```python
from build123d import *

# Parameters (mm, degrees)
F0_R     = 5
F1_DEPTH = 5
F0_R_2   = 10
F2_DEPTH = 15
F3_DEPTH = 10
F4_DEPTH = 5
F5_DEPTH = 20
F6_DEPTH = 10


with BuildPart() as f1:
    # F0 (on Front) → F1 (new body)
    with BuildSketch(Plane.XZ):
        with BuildLine():
            ThreePointArc((-20, 0), (-22.9289321881, 7.0710678119), (-30, 10))
            ThreePointArc((-30, 10), (-40, 0), (-30, -10))
            ThreePointArc((-30, -10), (-22.9289321881, -7.0710678119), (-20, 0))
        make_face()
        with Locations((-30, 0)):
            Circle(F0_R, mode=Mode.SUBTRACT)
    extrude(amount=F1_DEPTH)



with BuildPart() as f2:
    # F0 (on Front) → F2 (new body)
    with BuildSketch(Plane.XZ):
        with BuildLine():
            ThreePointArc((0, -15), (10.6066017178, -10.6066017178), (15, 0))
            ThreePointArc((15, 0), (10.6066017178, 10.6066017178), (0, 15))
            Line((0, 15), (-4.8648648649, 14.1891891892))
            ThreePointArc((-4.8648648649, 14.1891891892), (-15, 0), (-4.8648648649, -14.1891891892))
            Line((-4.8648648649, -14.1891891892), (0, -15))
        make_face()
        Circle(F0_R_2, mode=Mode.SUBTRACT)
    extrude(amount=F2_DEPTH)

    # F0 (on Front) → F3 (join)
    with BuildSketch(Plane.XZ):
        with BuildLine():
            ThreePointArc((50, 0), (45.6066017178, 10.6066017178), (35, 15))
            ThreePointArc((35, 15), (20, 0), (35, -15))
            ThreePointArc((35, -15), (45.6066017178, -10.6066017178), (50, 0))
        make_face()
        with Locations((35, 0)):
            Circle(F0_R_2, mode=Mode.SUBTRACT)
        with BuildLine():
            ThreePointArc((0, 15), (10.6066017178, 10.6066017178), (15, 0))
            ThreePointArc((15, 0), (10.6066017178, -10.6066017178), (0, -15))
            Line((0, -15), (35, -15))
            ThreePointArc((35, -15), (20, 0), (35, 15))
            Line((35, 15), (0, 15))
        make_face()
    extrude(amount=F3_DEPTH)

    # F0 (on Front) → F4 (join)
    with BuildSketch(Plane.XZ):
        with BuildLine():
            ThreePointArc((50, 0), (45.6066017178, 10.6066017178), (35, 15))
            ThreePointArc((35, 15), (20, 0), (35, -15))
            ThreePointArc((35, -15), (45.6066017178, -10.6066017178), (50, 0))
        make_face()
        with Locations((35, 0)):
            Circle(F0_R_2, mode=Mode.SUBTRACT)
        with BuildLine():
            ThreePointArc((0, 15), (10.6066017178, 10.6066017178), (15, 0))
            ThreePointArc((15, 0), (10.6066017178, -10.6066017178), (0, -15))
            Line((0, -15), (35, -15))
            ThreePointArc((35, -15), (20, 0), (35, 15))
            Line((35, 15), (0, 15))
        make_face()
    extrude(amount=-F4_DEPTH)

    # F0 (on Front) → F5 (join)
    with BuildSketch(Plane.XZ):
        with BuildLine():
            ThreePointArc((0, -15), (10.6066017178, -10.6066017178), (15, 0))
            ThreePointArc((15, 0), (10.6066017178, 10.6066017178), (0, 15))
            Line((0, 15), (-4.8648648649, 14.1891891892))
            ThreePointArc((-4.8648648649, 14.1891891892), (-15, 0), (-4.8648648649, -14.1891891892))
            Line((-4.8648648649, -14.1891891892), (0, -15))
        make_face()
        Circle(F0_R_2, mode=Mode.SUBTRACT)
    extrude(amount=-F5_DEPTH)


with BuildPart() as f1_1:
    add(f1.part)

    add(f2.part)  # F6 merges F2
    # F0 (on Front) → F6 (join)
    with BuildSketch(Plane.XZ):
        with BuildLine():
            ThreePointArc((-20, 0), (-22.9289321881, 7.0710678119), (-30, 10))
            ThreePointArc((-30, 10), (-40, 0), (-30, -10))
            ThreePointArc((-30, -10), (-22.9289321881, -7.0710678119), (-20, 0))
        make_face()
        with Locations((-30, 0)):
            Circle(F0_R, mode=Mode.SUBTRACT)
        with BuildLine():
            ThreePointArc((-4.8648648649, -14.1891891892), (-15, 0), (-4.8648648649, 14.1891891892))
            Line((-4.8648648649, 14.1891891892), (-30, 10))
            ThreePointArc((-30, 10), (-22.9289321881, 7.0710678119), (-20, 0))
            ThreePointArc((-20, 0), (-22.9289321881, -7.0710678119), (-30, -10))
            Line((-30, -10), (-4.8648648649, -14.1891891892))
        make_face()
    extrude(amount=-F6_DEPTH)


solid = f1_1.part
```
Input: part model. Units: mm. Frame: model coordinates. A direction names the side the tool comes from. Give positions to 0.01 mm unless a question says otherwise; leave off trailing zeros. Order: outer loops, then holes, each group sorted by start corner. A loop starts at its lowest first (then second) coordinate and runs counter-clockwise, first axis right, second up. Notation, with made-up numbers: M -15.5,29.25 L 26.5,29.25 A20 cw 26.5,61.25 Z; hole C 26.25,7.5 d11. An arc over 180 degrees is marked long. Return JSON: item names as keys, results as strings.
1) Section query C-C on z = 12. Output: boundary loops of the cut face in (x, y).
Taken from the geometry:
{"outline": "M -18,0 L -9,0 L -9,-15 L 9,-15 L 9,-10 L 44,-10 L 44,5 L 9,5 L 9,20 L -9,20 L -9,10 L -18,10 Z"}
2) Access query for faces 4 (the face through (15, -12, 0)), 5 (the face through (-15, -7, 0)), 6 (the face through (15, 12, 0)), 7 (the face through (-15, 15, 0)), 8 (the face through (-35, -5, -2)). Directions: +Z, -Z, +X, -X, +Y, -Y. A direction counts if a zero-diameter tool reaches every point of the face in a straight line with its end or side. Return the directions, or none.
Taken from the geometry:
{"face 4": "+X, -Y", "face 5": "-Y", "face 6": "+X, +Y", "face 7": "-X, +Y", "face 8": "+Z, -Z, -X, -Y"}
3) Line query: L1, parallel to Z at x = 35, y = 2; L2, parallel to Z at x = -30, y = -3.8; L3, parallel to X at y = 2.5, z = 3.5. Output: solid intervals per line, ascending. Write a range as [from, to].
Taken from the geometry:
{"L1": "z = [-15, -10], [10, 15]", "L2": "z = [-10, -5], [5, 10]", "L3": "x = [-39.37, -33.57], [-26.43, -9.37], [9.37, 25.63], [44.37, 49.59]"}
4) Section query A-A on y = -1.5. Output: boundary loops of the cut face in (x, z).
Taken from the geometry:
{"outline": "C -30,0 d20; M -4.86,-14.19 L 0,-15 L 35,-15 A15 ccw 35,15 L 0,15 L -4.86,14.19 A15 ccw Z; hole C -30,0 d10; hole C 0,0 d20; hole C 35,0 d20"}
5) Section query B-B on y = -6. Output: boundary loops of the cut face in (x, z).
Taken from the geometry:
{"outline": "M -4.86,-14.19 L 0,-15 L 35,-15 A15 ccw 35,15 L 0,15 L -4.86,14.19 A15 ccw Z; hole C 0,0 d20; hole C 35,0 d20"}
6) Mould query, pull axis Z, two halves, no side actions, for faces 1 (the face through (3, -15, -10)), 2 (the face through (17, -3, -15)), 3 (the face through (-2.17, 2.75, -9.76)). Classes: released by +Z, released by -Z, zero draft, split by the parting line, or undercut.
Taken from the geometry:
{"face 1": "zero draft", "face 2": "released by -Z", "face 3": "undercut"}
7) Section query D-D on x = 28.5. Output: boundary loops of the cut face in (y, z).
Taken from the geometry:
{"outline": "M -10,-15 L 5,-15 L 5,-7.6 L -10,-7.6 Z; M -10,7.6 L 5,7.6 L 5,15 L -10,15 Z"}
8) Contact query for flat-ended pins moving along their axis: pin 1 (3 mm diameter, centred on y = 8.5, z = 2.5, fed in from -X); pin 2 (1 mm diameter, centred on y = -11, z = 9.5, fed in from -X); pin 3 (1 mm diameter, centred on x = 26, z = 4, fed in from +Y); pin 4 (5 mm diameter, centred on x = 28.5, z = -1, fed in from +Y). Output: stop coordinate, or through.
Taken from the geometry:
{"pin 1": "stops at x = -39.95", "pin 2": "stops at x = -12", "pin 3": "stops at y = 5", "pin 4": "passes through"}
